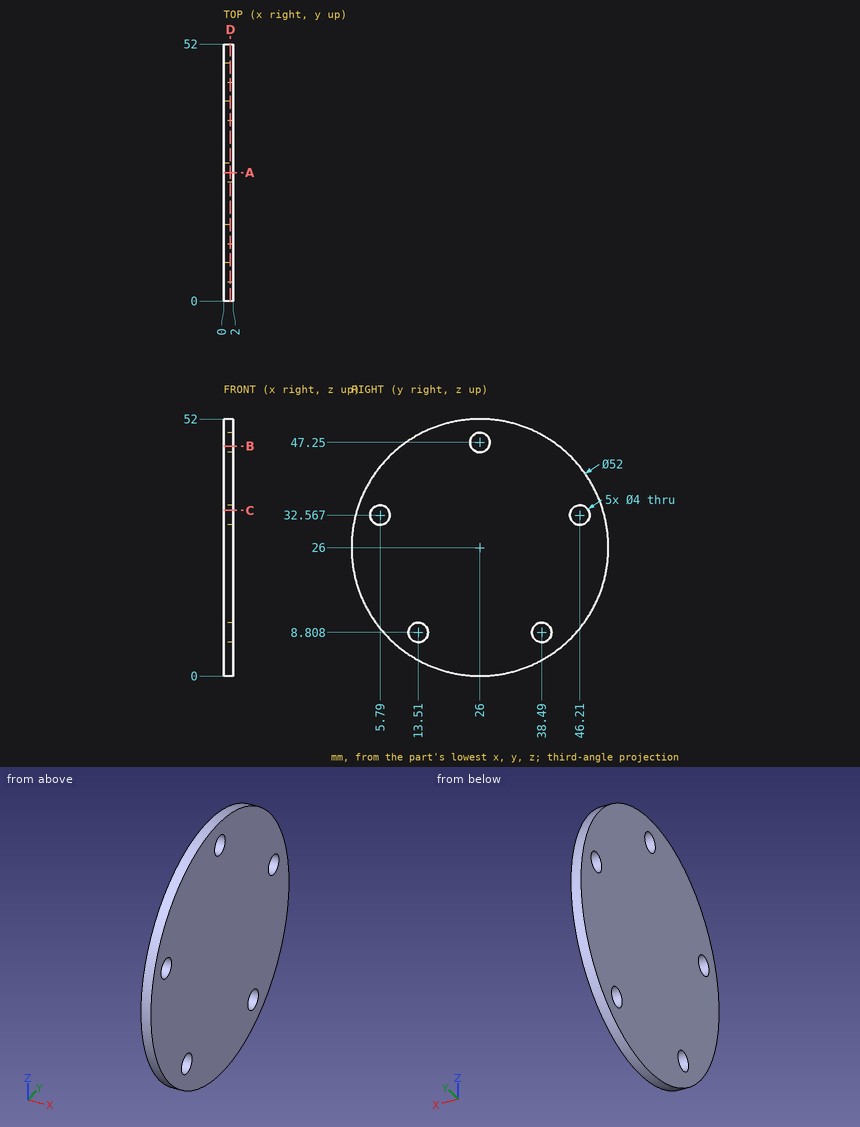
Geometry check sheet. Reference: drawing and pictorial views, mm from the part's lowest x, y, z. Give positions to 0.01 mm unless a question says otherwise; leave off trailing zeros. Loops run counter-clockwise (first coordinate to the right, second up) from the corner with the lowest first, then second, coordinate; pieces in that order, holes last. Notation, with made-up numbers: (77, 0.25) -> (86, 0.25) arc R30 ccw to (86, 25.25) -> close; hole circle Ø6 at (-23, 7). An arc over 180 degrees is marked (long way). Answer in a Markdown table with one row per item. Add a question column.
1) Cross-section at A-A on y = 26. Record the boundary of the cut face in (x, z).
2) Gauge pin test, flat ends, axial feed: P1, Ø1, axis at y = 47, z = 42.5, coming from the +X side; P2, Ø10, axis at y = 12.5, z = 28.5, coming from the -X side. Record the tip position at first contact, or that the pin passes through.
3) Cross-section at C-C on z = 33.5. Record the boundary of the cut face in (x, y) (1 decimal).
4) Cross-section at B-B on z = 46.5. Record the boundary of the cut face in (x, y).
5) Material ranges on probe 1 along Z at (x, y) = (0.55, 26); probe 2 along Y at (x, z) = (1.15, 31) (1 decimal); probe 3 along Y at (x, z) = (0.2, 12.5), recorded low to high. Write a range as from..to.
6) Cross-section at D-D on x = 1.4. Record the boundary of the cut face in (y, z), and give its area (3 significant figures).
Outcome:
| question | item | result |
|---|---|---|
| 1 | outline | (0, 0) -> (2, 0) -> (2, 45.25) -> (0, 45.25) -> close; (0, 49.25) -> (2, 49.25) -> (2, 52) -> (0, 52) -> close |
| 2 | P1 | passes through |
| 2 | P2 | stops at x = 0 |
| 3 | outline | (0, 1.1) -> (2, 1.1) -> (2, 4) -> (0, 4) -> close; (0, 7.6) -> (2, 7.6) -> (2, 44.4) -> (0, 44.4) -> close; (0, 48) -> (2, 48) -> (2, 50.9) -> (0, 50.9) -> close |
| 4 | outline | (0, 10.01) -> (2, 10.01) -> (2, 24.15) -> (0, 24.15) -> close; (0, 27.85) -> (2, 27.85) -> (2, 41.99) -> (0, 41.99) -> close |
| 5 | probe 1 | z = 0..45.25, 49.25..52 |
| 5 | probe 2 | y = 0.5..4.5, 7..45, 47.5..51.5 |
| 5 | probe 3 | y = 3.78..48.22 |
| 6 | outline | circle Ø52 at (26, 26); hole circle Ø4 at (5.79, 32.57); hole circle Ø4 at (13.51, 8.81); hole circle Ø4 at (26, 47.25); hole circle Ø4 at (38.49, 8.81); hole circle Ø4 at (46.21, 32.57) |
| 6 | area | 2,060 mm^2 |
